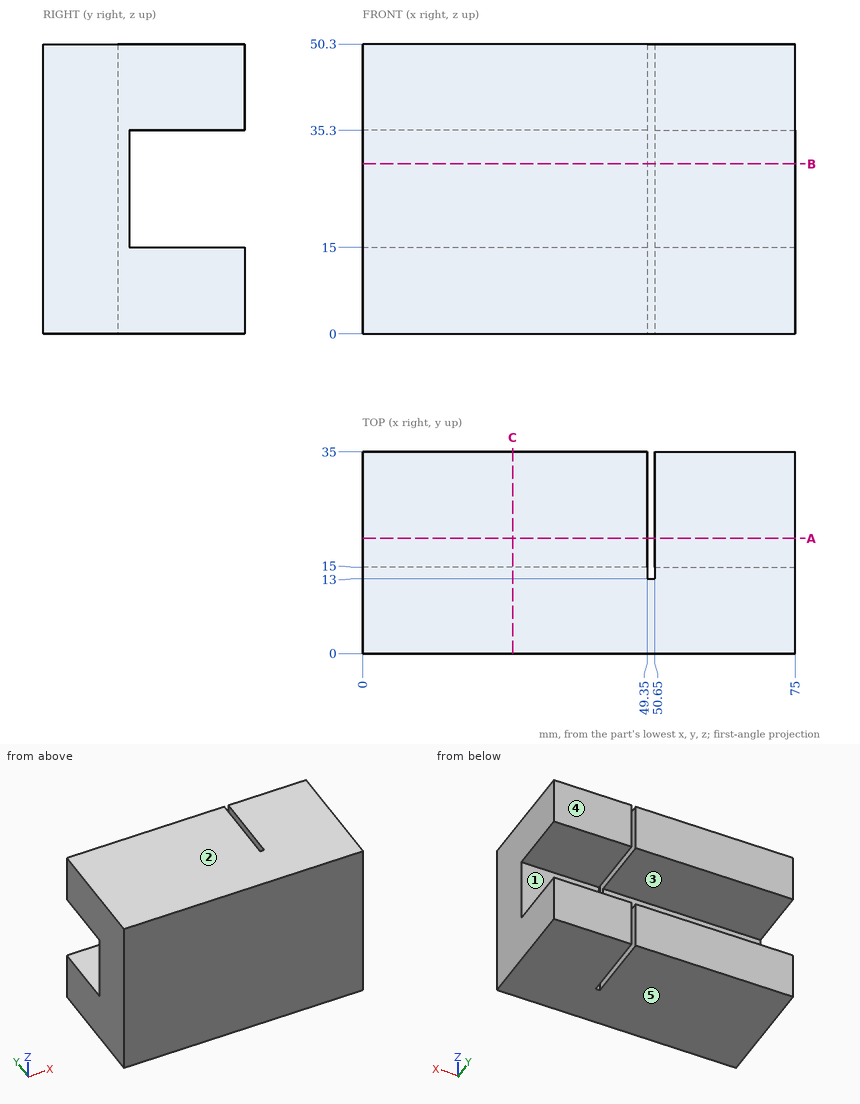
Source: three-view drawing plus pictorial views. Frame: mm from the lowest corner of the part. A direction names the side the tool comes from. Coordinates: 2 decimals unless noted, no trailing zeros. Order: outer loops, then holes, each group sorted by start corner. A loop starts at its lowest first (then second) coordinate and runs counter-clockwise, first axis right, second up. Notation, with made-up numbers: M 8,23 L 22,23 A33 ccw 22,54 Z; hole C 72.5,56.25 d9. An arc over 180 degrees is marked long. One line per question, with ' | ' between items. Start each with the question number.
Item 1: Draft query along Z for the marked faces 3, 4 and 5. Return one class per face: released by +Z, released by -Z, zero draft, split by the parting line, or undercut.
Item 2: Ray query, probe 1 along Z at (x, y) = (29.5, 21); probe 2 along X at (y, z) = (16, 6); probe 3 along Y at (x, z) = (70, 35). Return the intervals inside material, ascending. Write a range as [from, to].
Item 3: Pin query (flat end, axial travel): pin 1 Ø4 at (x, z) = (46, 27.5) entering from +Y. Return the tip coordinate at first contact, or that it passes through.
Item 4: Cut plane A-A, the plane y = 20. Return the cut outline in (x, z), then the cut area to 3 significant figures.
Item 5: Cut plane B-B, the plane z = 29.5. Return the cut outline in (x, y).
Item 6: Set-up query: the marked faces 1 and 2. Return all of +Z, -Z, +X, -X, +Y, -Y with unobstructed straight access to the full face (end or side cutting, diameter ignored); none if empty.
Item 7: Cut plane C-C, the plane x = 26. Return the cut outline in (y, z), then the cut area to 3 significant figures.
A:
1) face 3: undercut | face 4: zero draft | face 5: released by -Z
2) probe 1: z = [0, 15], [35.3, 50.3] | probe 2: x = [0, 49.35], [50.65, 75] | probe 3: y = [0, 15]
3) pin 1: stops at y = 15
4) outline: M 0,0 L 49.35,0 L 49.35,15 L 0,15 Z; M 0,35.3 L 49.35,35.3 L 49.35,50.3 L 0,50.3 Z; M 50.65,0 L 75,0 L 75,15 L 50.65,15 Z; M 50.65,35.3 L 75,35.3 L 75,50.3 L 50.65,50.3 Z | area: 2,210 mm2
5) outline: M 0,0 L 75,0 L 75,15 L 50.65,15 L 50.65,13 L 49.35,13 L 49.35,15 L 0,15 Z
6) face 1: +X, -X, +Y | face 2: +Z, +X, -X, +Y, -Y
7) outline: M 0,0 L 35,0 L 35,15 L 15,15 L 15,35.3 L 35,35.3 L 35,50.3 L 0,50.3 Z | area: 1,350 mm2
